Part model, mm, in its own coordinate system. Face numbers are marked on the shaded views. A direction names the side the tool comes from. Round coordinates to 2 decimals unless told otherwise and drop trailing zeros. Write each loop counter-clockwise with the first axis right and the second up, starting at its lowest first coordinate (ties: lowest second). Pieces come first, ordered by that corner, then holes. Notation, with made-up numbers: (67, 89) -> (87, 89) arc R19 ccw to (87, 98) -> close; hole circle Ø9 at (46.25, 67). An arc over 180 degrees is marked (long way). Return JSON: item names as keys, results as strings. Group by question number.
(1) Saw through at B-B (z = -10). List the corners of the cut face in (x, y), plus the area to 3 significant figures.
(2) Mould opens along Z. For the marked faces 1, 2 and 3 say: +Z half, -Z half, draft (parallel to the pull), parting line (faces both ways), or undercut.
(3) Saw through at A-A (x = 19). List the corners of the cut face in (y, z), plus the area to 3 significant figures.
(4) Saw through at D-D (x = 16). List the corners of the cut face in (y, z).
(5) Drop flat-ended pins along their axis: pin 1 Ø0.5 at (x, y) = (17, 2) entering from -Z; pin 2 Ø3 at (y, z) = (3.5, 1.5) entering from -X; pin 3 Ø1.6 at (x, y) = (11.5, 0.5) entering from +Z. Give the stop position or say it passes through.
(6) Tool access for the marked faces 4, 5 and 6: list every direction of +Z, -Z, +X, -X, +Y, -Y with a clear straight run to the whole face (end or side of a thin tool).
(7) Saw through at C-C (y = 2.75). List the corners of the cut face in (x, z).
(8) Drill centre lines: L1, parallel to X at y = 0.75, z = -10; L2, parallel to X at y = 4, z = 1.5; L3, parallel to Y at x = 5.75, z = 0. Where is each one in solid material? Low to high. Write a range as from..to.
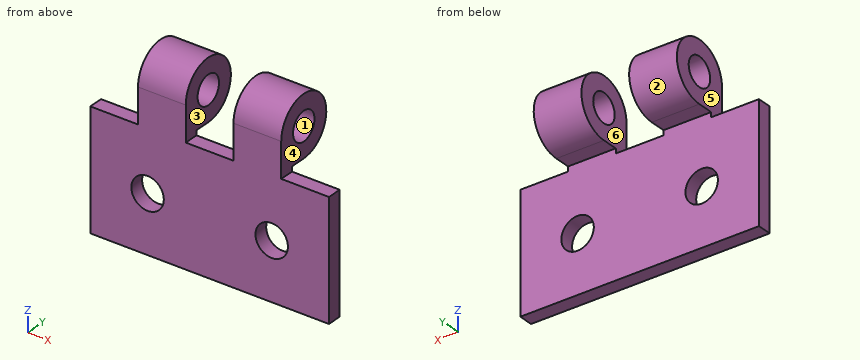
Autodesk Inventor part; units mm, degrees
ref_plane "1_XY" through (0, 3.15, 0) normal (1, 0, 0) x (0, 0, -1)
ref_plane "1_YZ" through (0, 3.15, 0) normal (0, 0, -1) x (0, 1, 0)
ref_plane "1_ZX" through (0, 3.15, 0) normal (0, 1, 0) x (1, 0, 0)
sketch "Sketch_10" plane through (0, 0, 0) normal (0, 1, 0) x (-1, 0, 0)
  line L0 (0, -3.65) -> (-5, -3.65)
  line L1 (-5, -3.65) -> (-5, -3.15)
  line L2 (-5, -3.15) -> (-10, -3.15)
  line L3 (-10, -3.15) -> (-10, -3.65)
  line L4 (-10, -3.65) -> (-15, -3.65)
  line L5 (-15, -3.65) -> (-15, -3.15)
  line L6 (-15, -3.15) -> (-20, -3.15)
  line L7 (-20, -3.15) -> (-20, -3.65)
  line L8 (-20, -3.65) -> (-25, -3.65)
  line L9 (-25, -3.65) -> (-25, -16)
  line L10 (-25, -16) -> (0, -16)
  line L11 (0, -16) -> (0, -3.65)
extrude "Extrusion1" add sketch "Sketch_10" along normal blind 1.5
sketch "Sketch_2" plane through (5, 0, 0) normal (1, 0, 0) x (0, 0, -1)
  arc A0 (3.15, 3.15) -> (0, 0) centre (0, 3.15) ccw
  line L0 (0, 0) -> (10.6667, 0)
  line L1 (10.6667, 0) -> (10.6667, 1.5)
  line L2 (10.6667, 1.5) -> (3.15, 1.5)
  line L3 (3.15, 1.5) -> (3.15, 3.15)
  circle A1 centre (0, 3.15) radius 1.5
extrude "Extrusion2" add sketch "Sketch_2" along normal blind 5
sketch "Sketch_3" plane through (15, 0, 0) normal (1, 0, 0) x (0, 0, -1)
  arc A0 (3.15, 3.15) -> (0, 0) centre (0, 3.15) ccw
  line L0 (0, 0) -> (10.6667, 0)
  line L1 (10.6667, 0) -> (10.6667, 1.5)
  line L2 (10.6667, 1.5) -> (3.15, 1.5)
  line L3 (3.15, 1.5) -> (3.15, 3.15)
  circle A1 centre (0, 3.15) radius 1.5
extrude "Extrusion3" add sketch "Sketch_3" along normal blind 5
sketch "Sketch4" plane through (0, 0, 0) normal (0, -1, 0) x (1, 0, 0)
  point P0 (6, -10)
hole "Hole1" at (6, 0, -10) direction (0, 1, 0) diameter 3.4 depth 2
sketch "Sketch5" plane through (0, 0, 0) normal (0, -1, 0) x (1, 0, 0)
  point P0 (19, -10)
hole "Hole2" at (19, 0, -10) direction (0, 1, 0) diameter 3.4 depth 2
ref_plane "1_XY" through (0, 3.15, 0) normal (1, 0, 0) x (0, 0, -1)
ref_plane "1_YZ" through (0, 3.15, 0) normal (0, 0, -1) x (0, 1, 0)
ref_plane "1_ZX" through (0, 3.15, 0) normal (0, 1, 0) x (1, 0, 0)
ref_plane "11_XY" through (0, 3.15, 0) normal (1, 0, 0) x (0, 0, -1)
ref_plane "11_YZ" through (0, 3.15, 0) normal (0, 0, -1) x (0, 1, 0)
ref_plane "11_ZX" through (0, 3.15, 0) normal (0, 1, 0) x (1, 0, 0)
properties part number "1HHKS25" material "ステンレス鋼"
Computed values:
{
 "1": {"outline": "(0, 0) -> (4.3, 0) -> (4.3, 1.5) -> (0, 1.5) -> close; (7.7, 0) -> (17.3, 0) -> (17.3, 1.5) -> (7.7, 1.5) -> close; (20.7, 0) -> (25, 0) -> (25, 1.5) -> (20.7, 1.5) -> close", "area": "27.3 mm2"},
 "2": {"face 1": "undercut", "face 2": "parting line", "face 3": "draft"},
 "3": {"outline": "(0, -16) -> (1.5, -16) -> (1.5, -11.7) -> (0, -11.7) -> close; (0, -8.3) -> (1.5, -8.3) -> (1.5, -3.15) -> (3.15, -3.15) arc R3.15 ccw (long way) to (0, 0) -> close; hole circle Ø3 at (3.15, 0)", "area": "40.4 mm2"},
 "4": {"outline": "(0, -16) -> (1.5, -16) -> (1.5, -3.15) -> (3.15, -3.15) arc R3.15 ccw (long way) to (0, 0) -> close; hole circle Ø3 at (3.15, 0)"},
 "5": {"pin 1": "z = -3.15", "pin 2": "x = 5", "pin 3": "z = -3.65"},
 "6": {"face 4": "+Z, +X, +Y, -Y", "face 5": "+Z, -X, +Y, -Y", "face 6": "+Z, +Y, -Y"},
 "7": {"outline": "(5, -3.15) -> (10, -3.15) -> (10, -1.45) -> (5, -1.45) -> close; (5, 1.45) -> (10, 1.45) -> (10, 3.12) -> (5, 3.12) -> close; (15, -3.15) -> (20, -3.15) -> (20, -1.45) -> (15, -1.45) -> close; (15, 1.45) -> (20, 1.45) -> (20, 3.12) -> (15, 3.12) -> close"},
 "8": {"L1": "0..4.3, 7.7..17.3, 20.7..25", "L2": "5..10, 15..20", "L3": "0..1.65, 4.65..6.3"}
}
